Autodesk Inventor part; units mm, degrees
ref_plane "YZ Plane" through (0, 0, 0) normal (1, 0, 0) x (0, 1, 0)
ref_plane "XZ Plane" through (0, 0, 0) normal (0, 1, 0) x (-1, 0, 0)
ref_plane "XY Plane" through (0, 0, 0) normal (0, 0, 1) x (1, 0, 0)
sketch "Sketch1" plane through (0, 0, 0) normal (0, 0, 1) x (1, 0, 0)
  circle A0 centre (0, 0) radius 2.25
  dimension "d0" = 4.5
extrude "Extrusion1" add sketch "Sketch1" along normal blind 1.5
fillet "Fillet1" radius 0.5 1 edges at (-2.25, 0, 0)
fillet "Fillet2" radius 1 1 edges at (-2.25, 0, 1.5)
sketch "Sketch2" plane through (0, 0, 1.5) normal (0, 0, 1) x (1, 0, 0)
  line L0 (1.675, 0.375) -> (1.675, -0.375)
  line L1 (-1.625, -0.375) -> (-1.625, 0.375)
  line L2 (-0.375, 1.625) -> (0.375, 1.625)
  line L3 (0.375, -1.675) -> (-0.375, -1.675)
  line L4 (-0.375, -1.675) -> (-0.375, -0.375)
  line L5 (-0.375, 0.375) -> (-0.375, 1.625)
  line L6 (-1.625, 0.375) -> (-0.375, 0.375)
  line L7 (0.375, 0.375) -> (1.675, 0.375)
  line L8 (0.375, 1.625) -> (0.375, 0.375)
  line L9 (0.375, -0.375) -> (0.375, -1.675)
  line L10 (1.675, -0.375) -> (0.375, -0.375)
  line L11 (-0.375, -0.375) -> (-1.625, -0.375)
  circle A0 centre (0, 0) radius 1.25
  dimension "d5" = 0.75
  dimension "d6" = 3.3
  dimension "d9" = 0.75
  dimension "d10" = 3.3
  dimension "d28" = 0.75
  dimension "d29" = 0.75
  dimension "d30" = 0.375
  dimension "d31" = 0.375
  dimension "d32" = 0.375
  dimension "d33" = 0.375
  dimension "d34" = 1.25
  dimension "d35" = 1.25
extrude "Extrusion2" cut sketch "Sketch2" against normal blind 1 contours L0 L10 A0 L7 | A0 L10 L9 L4 L11 L6 L5 L8 L7 | A0 L5 L2 L8 | L9 L3 L4 A0 | A0 L11 L1 L6
chamfer "Chamfer2" distance 0.25 angle 45 4 edges at (-0.375, 0.375, 1) (-0.375, -0.375, 1) (0.375, 0.375, 1) (0.375, -0.375, 1)
sketch "Sketch3" plane through (0, 0, 0) normal (0, 0, -1) x (-1, 0, 0)
  circle A0 centre (0, 0) radius 1.75
  circle A1 centre (0, 0) radius 1.25
  dimension "d19" = 2.5
extrude "Extrusion3" add sketch "Sketch3" along normal blind 5 contours A1
thread "Thread1"
chamfer "倒角3" distance 0.5 angle 45 4 edges at (-1.625, 0, 0.5) (0, 1.625, 0.5) (0, -1.675, 0.5) (1.675, 0, 0.5)
properties part number "screw_M3_5"
Here's how the part is built. I have some questions about the finished solid (model axes, mm). A direction names the side the tool comes from. Round coordinates to 2 decimals unless told otherwise and drop trailing zeros. Loops run counter-clockwise (first coordinate to the right, second up) from the corner with the lowest first, then second, coordinate; pieces in that order, holes last. Notation, with made-up numbers: (78.25, 79.5) - (104.25, 79.5) arc R12 ccw to (104.25, 93.5) - close; hole circle Ø1 at (-13.75, 23). An arc over 180 degrees is marked (long way). One line per question, with ' | ' between items. Start each with the question number.
Q1. Will these pins go through, and if not, where does the flat tip stop? pin 1 (0.8 mm diameter, centred on x = 1, z = 1, fed in from -Y); pin 2 (2 mm diameter, centred on x = -1.5, z = 0, fed in from +Y); pin 3 (1.5 mm diameter, centred on y = 1.5, z = 0.5, fed in from +X).
Q2. Please list where these lines run through material, in increasing order: line 1 (X direction, y = 0.55, z = -2); line 2 (Z direction, x = -0.55, y = -0.1); line 3 (Y direction, x = 1.15, z = 1.25) (3 decimals). Write a range as [from, to].
Q3. For faces 1 (the flat face through (1, -1, 0)), 2 (the flat face through (-0.375, 1, 1)), 3 (the flat face through (-0.7, 0.7, 1.5)), which set-ups out of +Z, -Z, +X, -X, +Y, -Y let a thin tool reach every point of the face, with its end or its side?
Q4. I want a section at C-C (z = -0.5). Write out the boundary of the cut face in (x, y), then the cut area to 3 significant figures.
Q5. We'd pull the mould along Y, two halves only. Please class faces 4 (the flat face through (1, -0.375, 1)), 5 (the cylindrical face through (0.27, 1.22, -2.46)), 6 (the flat face through (0, 0, -5)), 7 (the flat face through (0.375, 1, 1)): +Y half, -Y half, draft (parallel to the pull), parting line (faces both ways), or undercut.
Response values:
1) pin 1: stops at y = -2.11 | pin 2: stops at y = 2.16 | pin 3: stops at x = 2.12
2) line 1: x = [-1.12, 1.12] | line 2: z = [-5, 0.5] | line 3: y = [-1.527, -0.375], [0.375, 1.527]
3) face 1: -Z | face 2: +Z | face 3: +Z, +X, -X, +Y, -Y
4) outline: circle Ø2.5 at (0, 0) | area: 4.91 mm²
5) face 4: undercut | face 5: parting line | face 6: draft | face 7: undercut
